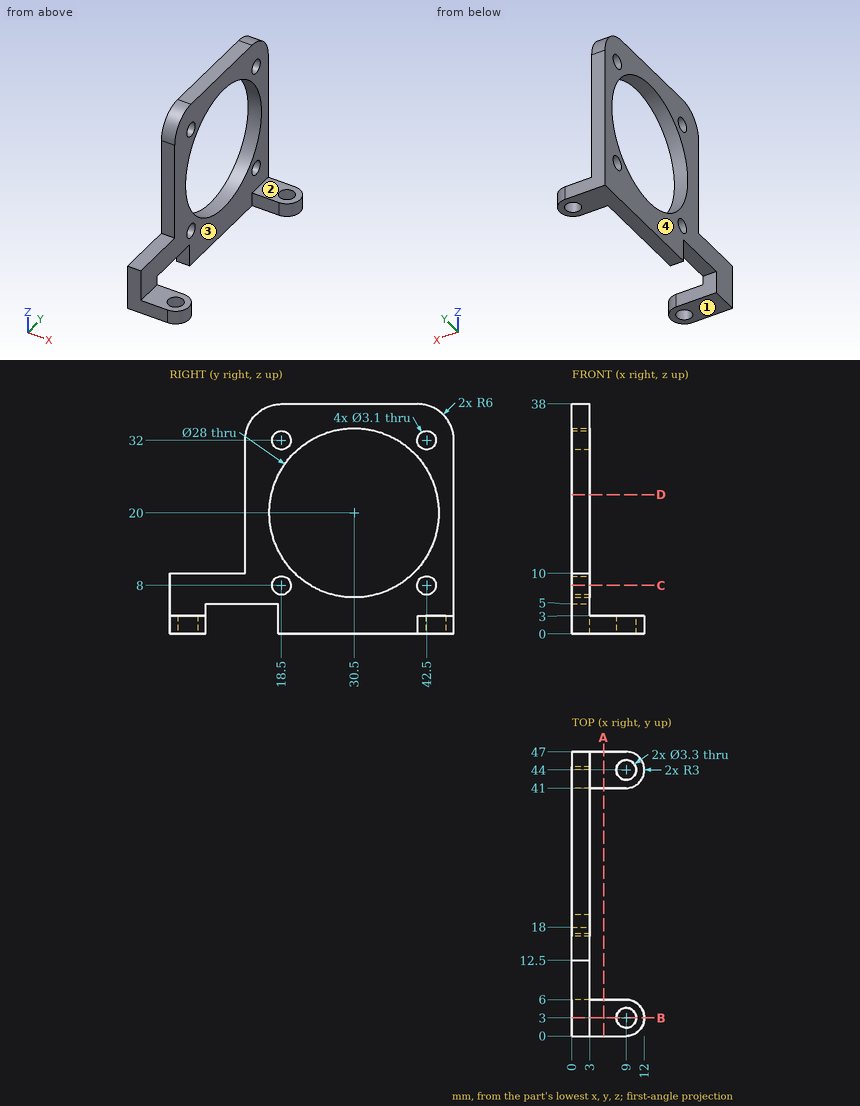
Geometry check sheet. Reference: drawing and pictorial views, mm from the part's lowest x, y, z. A direction names the side the tool comes from. Coordinates: 2 decimals unless noted, no trailing zeros. Order: outer loops, then holes, each group sorted by start corner. A loop starts at its lowest first (then second) coordinate and runs counter-clockwise, first axis right, second up. Notation, with made-up numbers: M -20,85 L 6,85 A17 cw 6,97 Z; hole C -16.75,75.5 d2. An arc over 180 degrees is marked long. Write each question's results on one line, items separated by ' | '. Start each with the question number.
1. Cross-section at B-B on y = 3. Record the cut outline in (x, z).
2. Cross-section at A-A on x = 5.25. Record the cut outline in (y, z).
3. Mould release check, pull along Y, two halves, no side actions. Record for the marked faces 3 and 4: +Y half, -Y half, draft (parallel to the pull), parting line (faces both ways), or undercut.
4. Material ranges on probe 1 along Y at (x, z) = (9, 2.05); probe 2 along Y at (x, z) = (2, 4.5); probe 3 along Y at (x, z) = (2.45, 8), recorded low to high.
5. Go/stop test with flat-tipped pins: P1, Ø2.5, axis at x = 2, y = 5, coming from the +Z side; P2, Ø6, axis at y = 21.5, z = 30, coming from the +X side; P3, Ø2, axis at x = 2, z = 7, coming from the -Y side; P4, Ø1.5, axis at x = 1, z = 21.5, coming from the -Y side. Record where each tip stops, or that it passes through.
6. Cross-section at C-C on z = 8. Record the cut outline in (x, y).
7. Access from +Z, -Z, +X, -X, +Y, -Y to the whole of each face (thin tool, end or side, straight path). Record for the marked faces 1 and 2.
8. Cross-section at D-D on z = 23. Record the cut outline in (x, y), and give its area (3 significant figures).
Checks:
1) outline: M 0,0 L 7.35,0 L 7.35,3 L 3,3 L 3,10 L 0,10 Z; M 10.65,0 L 12,0 L 12,3 L 10.65,3 Z
2) outline: M 0,0 L 6,0 L 6,3 L 0,3 Z; M 41,0 L 47,0 L 47,3 L 41,3 Z
3) face 3: undercut | face 4: draft
4) probe 1: y = 0 to 1.35, 4.65 to 6, 41 to 42.35, 45.65 to 47 | probe 2: y = 0 to 6, 18 to 47 | probe 3: y = 0 to 16.95, 20.05 to 23.29, 37.71 to 40.95, 44.05 to 47
5) P1: stops at z = 10 | P2: stops at x = 3 | P3: stops at y = 0 | P4: stops at y = 12.5
6) outline: M 0,0 L 3,0 L 3,16.95 L 0,16.95 Z; M 0,20.05 L 3,20.05 L 3,23.29 L 0,23.29 Z; M 0,37.71 L 3,37.71 L 3,40.95 L 0,40.95 Z; M 0,44.05 L 3,44.05 L 3,47 L 0,47 Z
7) face 1: -Z, +X, -X, +Y, -Y | face 2: +Z, +X, +Y, -Y
8) outline: M 0,12.5 L 3,12.5 L 3,16.83 L 0,16.83 Z; M 0,44.17 L 3,44.17 L 3,47 L 0,47 Z | area: 21.5 mm²
